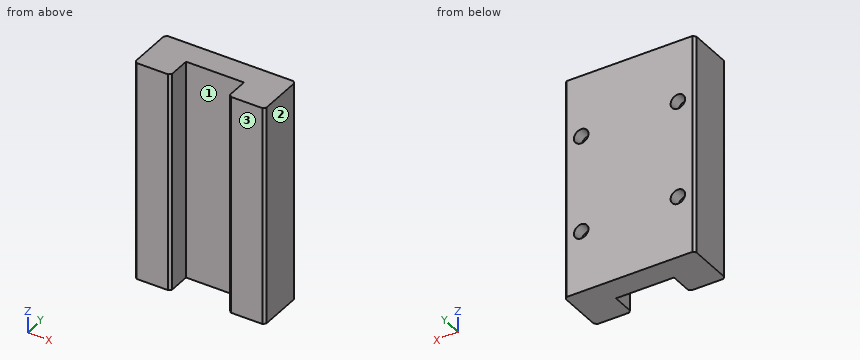
from build123d import *

# Parameters (mm, degrees)
EXTRUDE_1_DEPTH     = 45.4
SKETCH_2_R          = 1.5
CUT_EXTRUDE_1_DEPTH = 2.5
CHAMFER_1_SIZE      = 0.5


with BuildPart() as part:
    # 草图1 → 凸台-拉伸1 (new body)
    with BuildSketch(Plane.XY):
        Polygon((0, 0), (7.5, 0), (7.5, 5), (19.5, 5), (19.5, 0), (27, 0), (27, 10), (0, 10), align=None)
    extrude(amount=EXTRUDE_1_DEPTH)

    # 草图2 → 切除-拉伸1 (cut)
    with BuildSketch(Plane(origin=(0, 10, 0), x_dir=(1, 0, 0), z_dir=(0, 1, 0))):
        with Locations((23.5, -12.7)):
            Circle(SKETCH_2_R)
        with Locations((3.5, -12.7)):
            Circle(SKETCH_2_R)
        with Locations((23.5, -32.7)):
            Circle(SKETCH_2_R)
        with Locations((3.5, -32.7)):
            Circle(SKETCH_2_R)
    extrude(amount=-CUT_EXTRUDE_1_DEPTH, mode=Mode.SUBTRACT)

    # 倒角1
    chamfer_1_edges = [part.edges().sort_by_distance(p)[0] for p in [
        (0, 10, 22.7),
        (27, 10, 22.7),
        (27, 0, 22.7),
        (19.5, 0, 22.7),
        (7.5, 0, 22.7),
        (0, 0, 22.7),
    ]]
    chamfer(chamfer_1_edges, length=CHAMFER_1_SIZE)


solid = part.part
Model file for the job. Use its own axes, mm. Face numbers are marked on the shaded views. Give positions to 0.01 mm unless a question says otherwise; leave off trailing zeros. Order: outer loops, then holes, each group sorted by start corner. A loop starts at its lowest first (then second) coordinate and runs counter-clockwise, first axis right, second up. Notation, with made-up numbers: M -5.75,59 L 32.25,59 A33 cw 32.25,95 Z; hole C -13,89 d1. An arc over 180 degrees is marked long. Write item = value, one per line.
Q1. Cut at A-A, the plane y = 2.75. List the corners of the cut face in (x, z).
Derived:
outline = M 0,0 L 7.5,0 L 7.5,45.4 L 0,45.4 Z; M 19.5,0 L 27,0 L 27,45.4 L 19.5,45.4 Z
Q2. Drill centre lines: line 1 (Z direction, x = 3.5, y = 9.4); line 2 (X direction, y = 9.1, z = 12.7); line 3 (X direction, y = 3, z = 9.5). Where is each one in solid material? Low to high. Write a range as [from, to].
Derived:
line_1 = [0, 11.2], [14.2, 31.2], [34.2, 45.4]
line_2 = [0, 2], [5, 22], [25, 27]
line_3 = [0, 7.5], [19.5, 27]
Q3. Flat gauge pin, fed straight in: pin 1 (1.5 mm diameter, centred on x = 23.5, z = 12.5, fed in from +Y). Where does the tip first touch, or does it go through?
Derived:
pin_1 = 7.5
Q4. Cut at D-D, the plane z = 30.5. List the corners of the cut face in (x, y).
Derived:
outline = M 0,0.5 L 0.5,0 L 7,0 L 7.5,0.5 L 7.5,5 L 19.5,5 L 19.5,0.5 L 20,0 L 26.5,0 L 27,0.5 L 27,9.5 L 26.5,10 L 0.5,10 L 0,9.5 Z
Q5. Cut at B-B, the plane z = 12.7. List the corners of the cut face in (x, y).
Derived:
outline = M 0,0.5 L 0.5,0 L 7,0 L 7.5,0.5 L 7.5,5 L 19.5,5 L 19.5,0.5 L 20,0 L 26.5,0 L 27,0.5 L 27,9.5 L 26.5,10 L 25,10 L 25,7.5 L 22,7.5 L 22,10 L 5,10 L 5,7.5 L 2,7.5 L 2,10 L 0.5,10 L 0,9.5 Z
Q6. Two-plate mould, pull along X, no slides. Class the marked faces 1, 2 and 3: pulls with the +X half, pulls with the -X half, needs draft (parallel to the pull), parting line crosses it, or undercut.
Derived:
face_1 = undercut
face_2 = pulls with the +X half
face_3 = needs draft
Q7. Cut at C-C, the plane x = 23.5. List the corners of the cut face in (y, z).
Derived:
outline = M 0,0 L 10,0 L 10,11.2 L 7.5,11.2 L 7.5,14.2 L 10,14.2 L 10,31.2 L 7.5,31.2 L 7.5,34.2 L 10,34.2 L 10,45.4 L 0,45.4 Z
